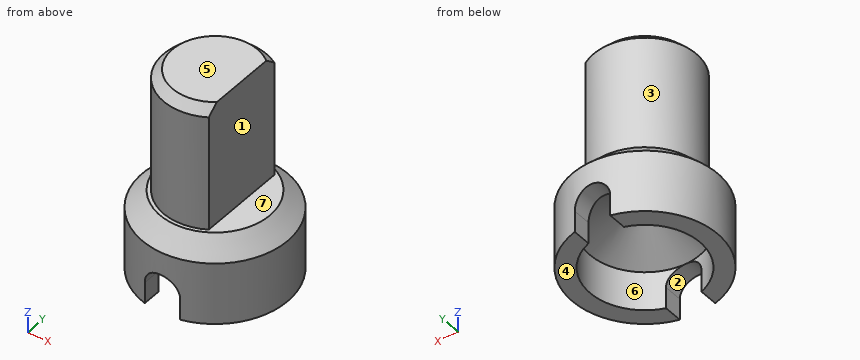
from build123d import *

# Parameters (mm, degrees)
F0_R     = 4.1
F1_DEPTH = 4.5
F2_D     = 6.2
F2_DEPTH = 2.2
F2_TIP   = 1.862667919
F4_DEPTH = 7
F5_SIZE  = 0.5
F6_SIZE  = 1
F8_DEPTH = 25


with BuildPart() as f1:
    # F0 (on Top) → F1 (new body)
    with BuildSketch(Plane.XY):
        Circle(F0_R)
    extrude(amount=F1_DEPTH)

    # F2
    with Locations(Plane(origin=(0, 0, 0), x_dir=(1, 0, 0), z_dir=(0, 0, -1))):
        with Locations((0, 0)):
            Hole(F2_D / 2, depth=F2_DEPTH)
            with Locations((0, 0, -(F2_DEPTH + F2_TIP / 2))):  # 118° drill point
                Cone(0, F2_D / 2, F2_TIP, mode=Mode.SUBTRACT)

    # F3 (on face) → F4 (join)
    with BuildSketch(Plane.XY.offset(4.5)):
        with BuildLine():
            Line((1.5, -2.4819347292), (1.5, 2.4819347292))
            ThreePointArc((1.5, 2.4819347292), (-2.9, 0), (1.5, -2.4819347292))
        make_face()
    extrude(amount=F4_DEPTH)

    # F5
    f5_edges = [f1.edges().sort_by_distance(p)[0] for p in [
        (-2.9, 0, 11.5),
    ]]
    chamfer(f5_edges, length=F5_SIZE)

    # F6
    f6_edges = [f1.edges().sort_by_distance(p)[0] for p in [
        (-4.1, 0, 4.5),
    ]]
    chamfer(f6_edges, length=F6_SIZE)

    # F7 (on Front) → F8 (cut, symmetric)
    with BuildSketch(Plane.XZ):
        with BuildLine():
            Line((-1, 1.2), (-1, 0))
            Line((-1, 0), (1, 0))
            Line((1, 0), (1, 1.2))
            ThreePointArc((1, 1.2), (0, 2.2), (-1, 1.2))
        make_face()
    extrude(amount=F8_DEPTH, both=True, mode=Mode.SUBTRACT)


solid = f1.part
Build history of the part. All positions in model axes, mm. Face numbers are marked on the shaded views. A direction names the side the tool comes from. Coordinates: 2 decimals unless noted, no trailing zeros. Order: outer loops, then holes, each group sorted by start corner. A loop starts at its lowest first (then second) coordinate and runs counter-clockwise, first axis right, second up. Notation, with made-up numbers: (6.5, 60) - (39.5, 60) arc R30 ccw to (39.5, 83) - close; hole circle Ø2 at (-0.75, -20). An arc over 180 degrees is marked (long way). Write each question's results on one line, items separated by ' | '. Start each with the question number.
Item 1: Band-saw the part on B-B on z = 2.75. Write the cut outline in (x, y).
Item 2: Band-saw the part on C-C on z = 10. Write the cut outline in (x, y), and give its area (3 significant figures).
Item 3: Mould opens along X. For the marked faces 1, 2, 3 and 4 say: released by +X, released by -X, zero draft, split by the parting line, or undercut.
Item 4: Flat gauge pins, fed straight in: pin 1 (1.5 mm diameter, centred on y = 3, z = 10, fed in from +X); pin 2 (1.1 mm diameter, centred on y = -3.5, z = 0.5, fed in from -X); pin 3 (1.5 mm diameter, centred on y = 2, z = 2, fed in from +X). Where does each tip first touch, or does it go through?
Item 5: Band-saw the part on A-A on z = 1.5. Write the cut outline in (x, y).
Item 6: Tool access for the marked faces 5, 6 and 7: list every direction of +Z, -Z, +X, -X, +Y, -Y with a clear straight run to the whole face (end or side of a thin tool).
Item 7: Wall check: probe 1 along Y at (x, z) = (-1.5, 5.5); probe 2 along X at (y, z) = (1.25, 3); probe 3 along Y at (x, z) = (0, 2.25). Give the ranges that are in metal, low to high. Write a range as [from, to].
Numbers:
1) outline: circle Ø8.2 at (0, 0); hole circle Ø4.37 at (0, 0)
2) outline: (1.5, -2.48) - (1.5, 2.48) arc R2.9 ccw (long way) to start | area: 21.5 mm^2
3) face 1: released by +X | face 2: undercut | face 3: split by the parting line | face 4: zero draft
4) pin 1: x = 1.5 | pin 2: x = -2.85 | pin 3: x = 3.9
5) outline: (-0.95, -3.99) - (-0.95, -2.95) arc R3.1 cw to (-0.95, 2.95) - (-0.95, 3.99) arc R4.1 ccw to start; (0.95, -3.99) arc R4.1 ccw to (0.95, 3.99) - (0.95, 2.95) arc R3.1 cw to (0.95, -2.95) - close
6) face 5: +Z, +X, -X, +Y, -Y | face 6: -Z | face 7: +Z
7) probe 1: [-2.48, 2.48] | probe 2: [-3.9, -1.25], [1.25, 3.9] | probe 3: [-4.1, -3.02], [3.02, 4.1]
